from build123d import *

# Parameters (mm, degrees)
BOSS_EXTRUDE1_DEPTH     = 18
CUT_EXTRUDE1_DEPTH      = 37.874680799
CUT_EXTRUDE1_DEPTH_BACK = 37.874680799
SKETCH2_R               = 2.5
SKETCH2_W               = 7
SKETCH2_H               = 23.578
SKETCH2_H_2             = 3
SKETCH3_R               = 2
CUT_EXTRUDE2_DEPTH      = 34.150597038
BOSS_EXTRUDE2_REACH     = 51.072
SKETCH4_W               = 7
SKETCH4_H               = 5


with BuildPart() as part:
    # Sketch1 → Boss-Extrude1 (new body)
    with BuildSketch(Plane.XY):
        Polygon((0, 0), (12.2, 0), (12.2, -28.578), (-14.8, -28.578), (-14.8, -23.578), (0, -23.578), align=None)
    extrude(amount=-BOSS_EXTRUDE1_DEPTH)

    # Sketch2 → Cut-Extrude1 (cut, two sides: drawn at the far end of the back side and taken through both)
    with BuildSketch(Plane.ZY.offset(-CUT_EXTRUDE1_DEPTH_BACK)):
        with Locations((-4.004934739, -20.578)):
            Circle(SKETCH2_R)
        with Locations((-4.004934739, -12.578)):
            Circle(SKETCH2_R)
        with Locations((-4.004934739, -4.578)):
            Circle(SKETCH2_R)
        with Locations((-14.5, -11.789)):
            Rectangle(SKETCH2_W, SKETCH2_H)
        with Locations((-3.5, -27.078)):
            Rectangle(SKETCH2_W, SKETCH2_H_2)
    extrude(amount=CUT_EXTRUDE1_DEPTH + CUT_EXTRUDE1_DEPTH_BACK, mode=Mode.SUBTRACT)

    # Sketch3 → Cut-Extrude2 (cut, through all)
    with BuildSketch(Plane(origin=(0, -23.578, 0), x_dir=(1, 0, 0), z_dir=(0, 1, 0))):
        with Locations(Location((-10.3, 3, 0), (0, 0, 270))):
            Circle(SKETCH3_R)
        with Locations(Location((6.1, 14.5, 0), (0, 0, 270))):
            Circle(SKETCH3_R)
    extrude(amount=-CUT_EXTRUDE2_DEPTH, mode=Mode.SUBTRACT)


with BuildPart() as body_2:
    # Mirror2: mirrored copy
    add(part.part.mirror(Plane(origin=(16.5, 0, 0), x_dir=(0, 0, 1), z_dir=(1, 0, 0))))

    # Sketch4 → Boss-Extrude2 (add, up to next)
    with BuildSketch(Plane(origin=(12.2, 0, 0), x_dir=(0, 0, -1), z_dir=(1, 0, 0)), mode=Mode.PRIVATE) as boss_extrude2_sk1:
        with Locations((14.5, -26.078)):
            Rectangle(SKETCH4_W, SKETCH4_H)
    boss_extrude2_tool1 = extrude(boss_extrude2_sk1.sketch, amount=BOSS_EXTRUDE2_REACH, mode=Mode.PRIVATE) - body_2.part

    add(part.part)  # Boss-Extrude2 merges part
    add(boss_extrude2_tool1.solids().sort_by_distance((12.2, -26.078, -14.5))[0])


solid = body_2.part
Geometry: final body of the model. Coordinates: model frame, mm. A direction names the side the tool comes from. Round coordinates to 2 decimals unless told otherwise and drop trailing zeros. Write each loop counter-clockwise with the first axis right and the second up, starting at its lowest first coordinate (ties: lowest second). Pieces come first, ordered by that corner, then holes. Notation, with made-up numbers: M -13,58.5 L 23,58.5 A21 cw 23,88.5 Z; hole C -28,60 d1. An arc over 180 degrees is marked long. Write item = value, one per line.
Item 1: Section query C-C on z = -14.5. Return loops of the section in (x, y), then the cut area to 3 significant figures.
Findings:
outline = M -14.8,-28.58 L 4.1,-28.58 L 4.1,-23.58 L -14.8,-23.58 Z; M 8.1,-28.58 L 24.9,-28.58 L 24.9,-23.58 L 8.1,-23.58 Z; M 28.9,-28.58 L 47.8,-28.58 L 47.8,-23.58 L 28.9,-23.58 Z
area = 273 mm^2
Item 2: Pull-direction query (X, two-part tool) for faces 5 (the face through (-1, -25.578, -4)), 6 (the face through (20.8, -14, -7)), 7 (the face through (0, -12, -7)); classes: pulls with the +X half, pulls with the -X half, needs draft (parallel to the pull), parting line crosses it, or undercut.
Findings:
face_5 = needs draft
face_6 = undercut
face_7 = pulls with the -X half
Item 3: Section query A-A on z = -8.5. Return loops of the section in (x, y).
Findings:
outline = M -14.8,-28.58 L 12.2,-28.58 L 12.2,0 L 0,0 L 0,-23.58 L -14.8,-23.58 Z; M 20.8,-28.58 L 47.8,-28.58 L 47.8,-23.58 L 33,-23.58 L 33,0 L 20.8,0 Z
Item 4: Material intervals for line 1 along X through (y, z) = (-24.05, -3); line 2 along X through (y, z) = (-1.5, -9); line 3 along Z through (x, y) = (26.9, -25.1), sorted ascending. Write a range as [from, to].
Findings:
line_1 = [-14.8, -12.3], [-8.3, 12.2], [20.8, 41.3], [45.3, 47.8]
line_2 = [0, 12.2], [20.8, 33]
line_3 = [-18, -16.5], [-12.5, 0]
Item 5: Access query for faces 1 (the face through (6, -12, -11)), 2 (the face through (33, -12, -7)), 3 (the face through (16, -26, -11)), 4 (the face through (16, -23.578, -13)). Directions: +Z, -Z, +X, -X, +Y, -Y. A direction counts if a zero-diameter tool reaches every point of the face in a straight line with its end or side. Return the directions, or none.
Findings:
face_1 = -Z, +X, -X, +Y
face_2 = +Z, -Z, +X, +Y
face_3 = +Z, +Y, -Y
face_4 = -Z, +Y
Item 6: Pin query (flat end, axial travel): P1, Ø1.5, axis at x = 15.5, y = -25.5, coming from the +Z side; P2, Ø12, axis at x = 38, y = -18, coming from the -Z side; P3, Ø13.5, axis at x = 4, y = -7, coming from the -Z side; P4, Ø5.5, axis at y = -7, z = -6.5, coming from the +X side. Return the tip coordinate at first contact, or that it passes through.
Findings:
P1 = -11
P2 = -18
P3 = -11
P4 = 33
Item 7: Section query B-B on x = 43.3. Return loops of the section in (y, z), then the cut area to 3 significant figures.
Findings:
outline = M -28.58,-18 L -23.58,-18 L -23.58,-5 L -25.58,-5 L -25.58,-7 L -28.58,-7 Z; M -25.58,-1 L -23.58,-1 L -23.58,0 L -25.58,0 Z
area = 61.0 mm^2
Item 8: Section query D-D on y = -17. Return loops of the section in (x, z).
Findings:
outline = M 0,-11 L 12.2,-11 L 12.2,0 L 0,0 Z; M 20.8,-11 L 33,-11 L 33,0 L 20.8,0 Z
